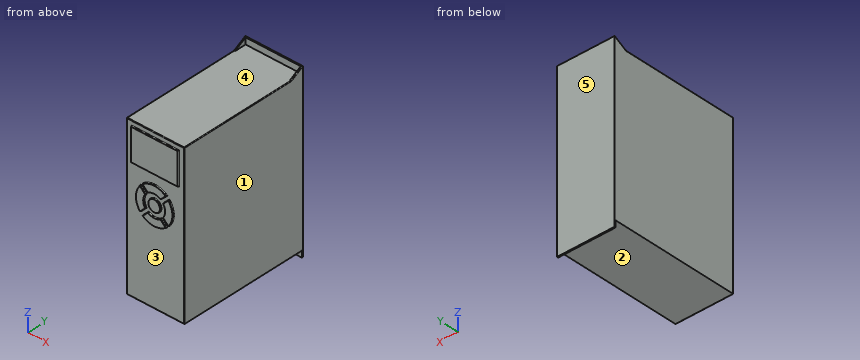
```python
from build123d import *

# Parameters (mm, degrees)
F0_W      = 90
F0_H      = 248
F1_DEPTH  = 205
F2_W      = 90
F2_H      = 248
F2_R      = 9
F2_W_2    = 73.0899348855
F2_H_2    = 49.802608788
F3_DEPTH  = 2
F4_W      = 90
F4_H      = 10
F5_DEPTH  = 20
F7_DEPTH  = 10
F9_DEPTH  = 90.001
F10_R     = 1
F11_DEPTH = 18


with BuildPart() as f1:
    # F0 (on Front) → F1 (new body)
    with BuildSketch(Plane.XZ):
        Rectangle(F0_W, F0_H)
    extrude(amount=F1_DEPTH)

    # F2 (on face) → F3 (cut)
    with BuildSketch(Plane.XZ.offset(205)):
        Rectangle(F2_W, F2_H)
        with BuildLine():
            ThreePointArc((-22.1542112523, 4.0888261413), (-28.4888623982, 21.9367015102), (-22.2335868368, 39.8125508039))
            Line((-22.2335868368, 39.8125508039), (-14.0800879143, 31.6590518814))
            ThreePointArc((-14.0800879143, 31.6590518814), (-17.0746019847, 21.9360306146), (-14.0073171141, 12.2357202795))
            Line((-14.0073171141, 12.2357202795), (-22.1542112523, 4.0888261413))
        make_face(mode=Mode.SUBTRACT)
        with BuildLine():
            Line((9.659050138, 7.9199138292), (17.8125490605, -0.2335850934))
            ThreePointArc((17.8125490605, -0.2335850934), (-0.0635810751, -6.4888600293), (-17.9116123889, -0.1538563696))
            Line((-17.9116123889, -0.1538563696), (-9.7647469179, 7.9930091015))
            ThreePointArc((-9.7647469179, 7.9930091015), (-0.0642548211, 4.9254008239), (9.659050138, 7.9199138292))
        make_face(mode=Mode.SUBTRACT)
        with BuildLine():
            ThreePointArc((-18.0098373075, 44.0740826489), (-0.0635511695, 50.4888635829), (17.9111756021, 44.1542129957))
            Line((17.9111756021, 44.1542129957), (9.7642814639, 36.0073188576))
            ThreePointArc((9.7642814639, 36.0073188576), (-0.0641690046, 39.0746029857), (-9.8692875132, 35.9335328546))
            Line((-9.8692875132, 35.9335328546), (-18.0098373075, 44.0740826489))
        make_face(mode=Mode.SUBTRACT)
        with Locations((0, 22.0000017434)):
            Circle(F2_R, mode=Mode.SUBTRACT)
        with BuildLine():
            ThreePointArc((22.153858113, 39.9116141324), (28.4888624646, 21.9367314157), (22.0740809054, 3.990164436))
            Line((22.0740809054, 3.990164436), (13.9335311111, 12.1307142303))
            ThreePointArc((13.9335311111, 12.1307142303), (17.074602306, 21.936116431), (14.006992642, 31.7647486613))
            Line((14.006992642, 31.7647486613), (22.153858113, 39.9116141324))
        make_face(mode=Mode.SUBTRACT)
        with Locations((0.1340024173, 91.3970731199)):
            Rectangle(F2_W_2, F2_H_2, mode=Mode.SUBTRACT)
    extrude(amount=-F3_DEPTH, mode=Mode.SUBTRACT)

    # F4 (on face) → F5 (join)
    with BuildSketch(Plane(origin=(0, 0, 0), x_dir=(-1, 0, 0), z_dir=(0, 1, 0))):
        with Locations((0, 129)):
            Rectangle(F4_W, F4_H)
        with Locations((0, -129)):
            Rectangle(F4_W, F4_H)
    extrude(amount=-F5_DEPTH)

    # F6 (on face) → F7 (cut, through all)
    with BuildSketch(Plane.XY.offset(134)):
        Polygon((43, -2), (-43, -2), (-43, -20), (43, -20), (43, -18), align=None)
    extrude(amount=-F7_DEPTH, mode=Mode.SUBTRACT)

    # F8 (on face) → F9 (cut, through all)
    with BuildSketch(Plane.YZ.offset(45)):
        Polygon((-20, 134), (-20, 124), (-2, 134), align=None)
    extrude(amount=-F9_DEPTH, mode=Mode.SUBTRACT)

    # F10
    f10_edges = [f1.edges().sort_by_distance(p)[0] for p in [
        (-45, -111.5, 124),
        (-45, -11, 129),
        (45, -11, 129),
        (45, -111.5, 124),
        (0, -203, -124),
        (45, -203, 0),
        (0, -203, 124),
        (-45, -203, 0),
        (-18.156837, -203, 35.735801),
        (-17.074602, -203, 21.936031),
        (-18.080764, -203, 8.162273),
        (-28.488862, -203, 21.936702),
        (-0.064255, -203, 4.925401),
        (13.7358, -203, 3.843164),
        (-0.063581, -203, -6.48886),
        (-13.83818, -203, 3.919576),
        (-0.064169, -203, 39.074603),
        (-13.939562, -203, 40.003808),
        (-0.063551, -203, 50.488864),
        (13.837729, -203, 40.080766),
        (-9, -203, 22.000002),
        (28.488862, -203, 21.936731),
        (18.003806, -203, 8.060439),
        (17.074602, -203, 21.936116),
        (18.080425, -203, 35.838181),
        (-36.410965, -203, 91.397073),
        (0.134002, -203, 116.298378),
        (36.67897, -203, 91.397073),
        (0.134002, -203, 66.495769),
    ]]
    fillet(f10_edges, radius=F10_R)

    # F11 (cut): a face of the model
    f11_faces = [f1.faces().sort_by_distance(p)[0] for p in [
        (0, -20, -129),
    ]]
    extrude(f11_faces, amount=-F11_DEPTH, mode=Mode.SUBTRACT)


solid = f1.part
```
CAD build for the part. Positions are in the model's coordinates, mm. Face numbers are marked on the shaded views. A direction names the side the tool comes from. Round coordinates to 2 decimals unless told otherwise and drop trailing zeros. Order: outer loops, then holes, each group sorted by start corner. A loop starts at its lowest first (then second) coordinate and runs counter-clockwise, first axis right, second up. Notation, with made-up numbers: (19, 17.5) - (62, 17.5) arc R26 cw to (62, 42.5) - close; hole circle Ø1 at (35, 29). An arc over 180 degrees is marked (long way). Answer in a Markdown table with one row per item. Add a question column.
(1) Band-saw the part on A-A on y = -147. List the corners of the cut face in (x, z), and give its area (3 significant figures).
(2) Drop flat-ended pins along their axis: pin 1 Ø8 at (x, y) = (-26, -39) entering from -Z; pin 2 Ø10 at (x, z) = (-1.5, -18.5) entering from -Y; pin 3 Ø0.5 at (y, z) = (-204.5, 82.5) entering from +X. Give the stop position or say it passes through.
(3) Mould opens along Z. For the marked faces 3, 4 and 5 say: +Z half, -Z half, draft (parallel to the pull), parting line (faces both ways), or undercut.
(4) Probe L1, parallel to Z at x = -20, y = -163.5; L2, parallel to Y at x = -8.5, z = -94; L3, parallel to X at y = -30, z = 123.5. List the from-to ranges inside material, lowest first. Write a range as [from, to].
(5) 3-axis set-ups, long thin cutter, end or side, ignore diameter. For the marked faces 1 and 2: which of +Z, -Z, +X, -X, +Y, -Y reach the whole face in a straight line?
Data:
| question | item | result |
|---|---|---|
| 1 | outline | (-45, -124) - (45, -124) - (45, 123) arc R1 ccw to (44, 124) - (-44, 124) arc R1 ccw to (-45, 123) - close |
| 1 | area | 22,300 mm^2 |
| 2 | pin 1 | stops at z = -124 |
| 2 | pin 2 | stops at y = -203 |
| 2 | pin 3 | stops at x = 36.68 |
| 3 | face 3 | undercut |
| 3 | face 4 | +Z half |
| 3 | face 5 | draft |
| 4 | L1 | z = [-124, 124] |
| 4 | L2 | y = [-203, 0] |
| 4 | L3 | x = [-44.87, 44.87] |
| 5 | face 1 | +Z, -Z, +X, +Y, -Y |
| 5 | face 2 | -Z, +X, -X, -Y |
